```python
from build123d import *

# Parameters (mm, degrees)
EXTRUDE_1_DEPTH = 50


with BuildPart() as part:
    # 스케치1 → 보스-돌출1 (new body)
    with BuildSketch(Plane(origin=(0, 0, 0), x_dir=(0, 0, -1), z_dir=(1, 0, 0))):
        with BuildLine():
            Line((-68.041278197, 50.714063441), (373.078721803, 230.214063441))
            ThreePointArc((373.078721803, 230.214063441), (442.026414912, 205.264519299), (424.332130863, 134.108518499))
            Line((424.332130863, 134.108518499), (158.212130863, -45.391481501))
            ThreePointArc((158.212130863, -45.391481501), (143.603146836, -52.359602267), (127.595225221, -54.752))
            Line((127.595225221, -54.752), (-47.404774779, -54.752))
            ThreePointArc((-47.404774779, -54.752), (-101.137808871, -10.513921782), (-68.041278197, 50.714063441))
        make_face()
        with BuildLine():
            Line((-66.250208204, 46.312521406), (374.869791796, 225.812521406))
            ThreePointArc((374.869791796, 225.812521406), (437.833421534, 203.028381884), (421.674848287, 138.048106461))
            Line((421.674848287, 138.048106461), (155.554848287, -41.451893539))
            ThreePointArc((155.554848287, -41.451893539), (142.213797707, -47.815241696), (127.595225221, -50))
            Line((127.595225221, -50), (-47.404774779, -50))
            ThreePointArc((-47.404774779, -50), (-96.474246298, -9.601404316), (-66.250208204, 46.312521406))
        make_face(mode=Mode.SUBTRACT)
    extrude(amount=EXTRUDE_1_DEPTH)


solid = part.part
```
The listing builds one solid part. Answer for the finished solid, in the listing's coordinates (mm). A direction names the side the tool comes from. Round coordinates to 2 decimals unless told otherwise and drop trailing zeros. Loops run counter-clockwise (first coordinate to the right, second up) from the corner with the lowest first, then second, coordinate; pieces in that order, holes last.
Q1. Section C-C, the plane y = 215 is taken. Determine the outline of the cut face in (x, z).
Q2. Section B-B, the plane z = -294 is taken. Determine the outline of the cut face in (x, y).
Q3. Find the intervals of material crossed by line 1 (Z direction, x = 38, y = 163.5); line 2 (Y direction, x = 11, z = -417.5); line 3 (Z direction, x = 45.5, y = 154), in increasing order.
Q4. For a pull along Y with two mould halves and no side action, classify faces 1 (the face through (24.65, 49.555, -290.478)), 2 (the face through (50, 155, -195)), 3 (the face through (24.65, 139.208, -149.431)), 4 (the face through (24.65, -47.754, -142.412)) as released by +Y, released by -Y, zero draft, split by the parting line, or undercut.
Q5. Given pin 1 Ø5 at (x, y) = (5.5, 105.5) entering from +Z; pin 2 Ø3 at (x, y) = (26.5, 13.5) entering from +Z; pin 3 Ø8 at (x, z) = (5.5, -139) entering from -Y, each flat-ended and moving along its own axis, determine where each tip first touches the part or whether it passes through.
Q6. Section A-A, the plane x = 34 is taken. Determine the outline of the cut face in (y, z), then the cut area to 3 significant figures.
Q7. Which of the six approach directions +Z, -Z, +X, -X, +Y, -Y give full straight-line access (tool end or side, diameter ignored) to faces 5 (the face through (25, -54.752, -41)), 6 (the face through (24.65, -10.55, 96.28))?
Completed:
1. outline: (0, -435.4) - (50, -435.4) - (50, -428.93) - (0, -428.93) - close; (0, -348.3) - (50, -348.3) - (50, -335.69) - (0, -335.69) - close
2. outline: (0, 46.2) - (50, 46.2) - (50, 51.93) - (0, 51.93) - close; (0, 192.91) - (50, 192.91) - (50, 198.04) - (0, 198.04) - close
3. line 1: z = -446.08 to -441.09, -221.74 to -209.13
3. line 2: y = 129.5 to 135.23, 223.48 to 228.82
3. line 3: z = -442.17 to -436.72, -198.39 to -185.78
4. face 1: undercut
4. face 2: zero draft
4. face 3: released by +Y
4. face 4: undercut
5. pin 1: stops at z = -60.45
5. pin 2: stops at z = 100.83
5. pin 3: stops at y = -54.25
6. outline: (-54.75, -127.6) arc R54.75 ccw to (-45.39, -158.21) - (134.11, -424.33) arc R54.75 ccw to (230.21, -373.08) - (50.71, 68.04) arc R54.75 ccw to (-54.75, 47.4) - close; hole (-50, -127.6) arc R50 ccw to (-41.45, -155.55) - (138.05, -421.67) arc R50 ccw to (225.81, -374.87) - (46.31, 66.25) arc R50 ccw to (-50, 47.4) - close
6. area: 6,180 mm2
7. face 5: +Z, -Z, +X, -X, -Y
7. face 6: +X, -X
